Autodesk Inventor part; units mm, degrees
ref_plane "YZ Plane" through (0, 0, 0) normal (1, 0, 0) x (0, 1, 0)
ref_plane "XZ Plane" through (0, 0, 0) normal (0, 1, 0) x (-1, 0, 0)
ref_plane "XY Plane" through (0, 0, 0) normal (0, 0, 1) x (1, 0, 0)
sketch "Skizze1" plane through (0, 0, 0) normal (0, 1, 0) x (-1, 0, 0)
  line L0 (-27.5, -16.25) -> (27.5, -16.25)
  line L1 (27.5, -16.25) -> (27.5, 16.25)
  line L2 (27.5, 16.25) -> (-27.5, 16.25)
  line L3 (-27.5, 16.25) -> (-27.5, -16.25)
  line L4 (-38.5, 0) -> (38.5, 0)
  line L5 (0, -22.75) -> (0, 22.75)
  point P0 (0, 0)
  dimension "d0" = 55
  dimension "d1" = 32.5
extrude "Extrusion1" add sketch "Skizze1" along normal blind 5
sketch "Skizze5" plane through (0, 5, 0) normal (0, 1, 0) x (1, 0, 0)
  line L0 (27.5, 16.25) -> (-27.5, 16.25)
  line L1 (27.5, -16.25) -> (27.5, 16.25)
  line L2 (-27.5, 16.25) -> (27.5, 16.25)
  line L3 (27.5, 16.25) -> (27.5, -16.25)
  line L4 (27.5, -16.25) -> (-27.5, -16.25)
  line L5 (-27.5, -16.25) -> (-27.5, 16.25)
  line L6 (-25.5, 14.25) -> (25.5, 14.25)
  line L7 (25.5, 14.25) -> (25.5, -14.25)
  line L8 (25.5, -14.25) -> (-25.5, -14.25)
  line L9 (-25.5, -14.25) -> (-25.5, 14.25)
  point P0 (0, 0)
  dimension "d14" = 2
extrude "Extrusion5" add sketch "Skizze5" along normal blind 10
sketch "Skizze6" plane through (0, 5, 0) normal (0, 1, 0) x (1, 0, 0)
  circle A0 centre (0, 0) radius 6
  circle A1 centre (0, 0) radius 7
  dimension "d17" = 12
  dimension "d18" = 14
extrude "Extrusion6" add sketch "Skizze6" along normal blind 2
extrude "Extrusion7" add sketch "Skizze6" along normal blind 12 contours A0
sketch "Skizze8" plane through (0, 17, 0) normal (0, 1, 0) x (1, 0, 0)
  circle A0 centre (0, 0) radius 3.95
  dimension "d23" = 7.9
extrude "Extrusion8" add sketch "Skizze8" along normal blind 2
sketch "Skizze9" plane through (0, 19, 0) normal (0, 1, 0) x (1, 0, 0)
  circle A0 centre (0, 0) radius 2
  dimension "d26" = 4
extrude "Extrusion9" cut sketch "Skizze9" against normal blind 4
properties part number "Servoverbindung_Konzept"
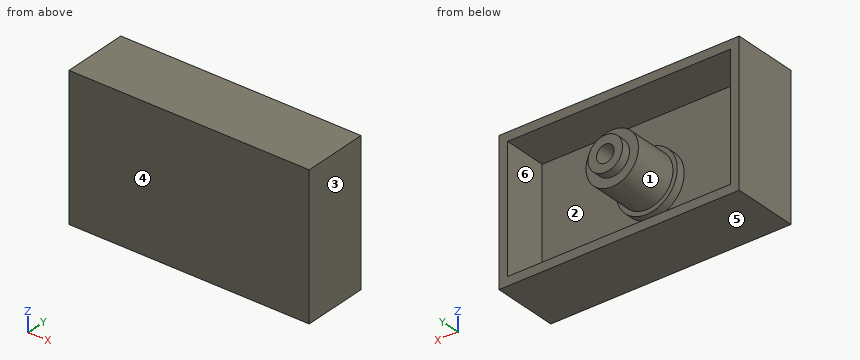
Build history of the part. All positions in model axes, mm. Face numbers are marked on the shaded views. A direction names the side the tool comes from. Round coordinates to 2 decimals unless told otherwise and drop trailing zeros. Write each loop counter-clockwise with the first axis right and the second up, starting at its lowest first coordinate (ties: lowest second). Pieces come first, ordered by that corner, then holes. Notation, with made-up numbers: M 56,80.5 L 104,80.5 A36 cw 104,119.5 Z; hole C 47.25,15.5 d11. An arc over 180 degrees is marked long. Answer as a JSON object with one key per item and string values. Group by question number.
(1) Drill centre lines: L1, parallel to X at y = 11.25, z = -13.5; L2, parallel to X at y = 17.15, z = 0; L3, parallel to Z at x = -14.5, y = 8.5. Where is each one in solid material? Low to high.
(2) Cut at C-C (x = 0). Give the cut face in (y, z).
(3) Cut at B-B (z = 0). Give the cut face in (x, y).
(4) Flat gauge pins, fed straight in: pin 1 (2.5 mm diameter, centred on x = 0, z = 0, fed in from +Y); pin 2 (1 mm diameter, centred on x = 5, z = 0, fed in from +Y). Where does each tip first touch, or does it go through?
(5) Cut at D-D (y = 12). Give the cut face in (x, z).
(6) Mould opens along X. For the marked faces 1, 2, 3 and 4 say: pulls with the +X half, pulls with the -X half, needs draft (parallel to the pull), parting line crosses it, or undercut.
(7) Which spindle directions (+Z, -Z, +X, -X, +Y, -Y) get a long thin tool onto all of the face, cutting with end or side? Do the marked faces 5 and 6. Say none if no direction does.
(8) Cut at A-A (y = 6). Give the cut face in (x, z), and give its area (3 significant figures).
Responses:
{
 "1": {"L1": "x = -27.5 to -25.5, 25.5 to 27.5", "L2": "x = -3.95 to -2, 2 to 3.95", "L3": "z = -16.25 to -14.25, 14.25 to 16.25"},
 "2": {"outline": "M 0,-16.25 L 15,-16.25 L 15,-14.25 L 5,-14.25 L 5,-7 L 7,-7 L 7,-6 L 17,-6 L 17,-3.95 L 19,-3.95 L 19,-2 L 15,-2 L 15,2 L 19,2 L 19,3.95 L 17,3.95 L 17,6 L 7,6 L 7,7 L 5,7 L 5,14.25 L 15,14.25 L 15,16.25 L 0,16.25 Z"},
 "3": {"outline": "M -27.5,0 L 27.5,0 L 27.5,15 L 25.5,15 L 25.5,5 L 7,5 L 7,7 L 6,7 L 6,17 L 3.95,17 L 3.95,19 L 2,19 L 2,15 L -2,15 L -2,19 L -3.95,19 L -3.95,17 L -6,17 L -6,7 L -7,7 L -7,5 L -25.5,5 L -25.5,15 L -27.5,15 Z"},
 "4": {"pin 1": "stops at y = 15", "pin 2": "stops at y = 17"},
 "5": {"outline": "M -27.5,-16.25 L 27.5,-16.25 L 27.5,16.25 L -27.5,16.25 Z; C 0,0 d12; hole M -25.5,-14.25 L 25.5,-14.25 L 25.5,14.25 L -25.5,14.25 Z"},
 "6": {"face 1": "undercut", "face 2": "undercut", "face 3": "pulls with the +X half", "face 4": "needs draft"},
 "7": {"face 5": "-Z, +X, -X, +Y, -Y", "face 6": "+Y"},
 "8": {"outline": "M -27.5,-16.25 L 27.5,-16.25 L 27.5,16.25 L -27.5,16.25 Z; C 0,0 d14; hole M -25.5,-14.25 L 25.5,-14.25 L 25.5,14.25 L -25.5,14.25 Z", "area": "488 mm2"}
}
